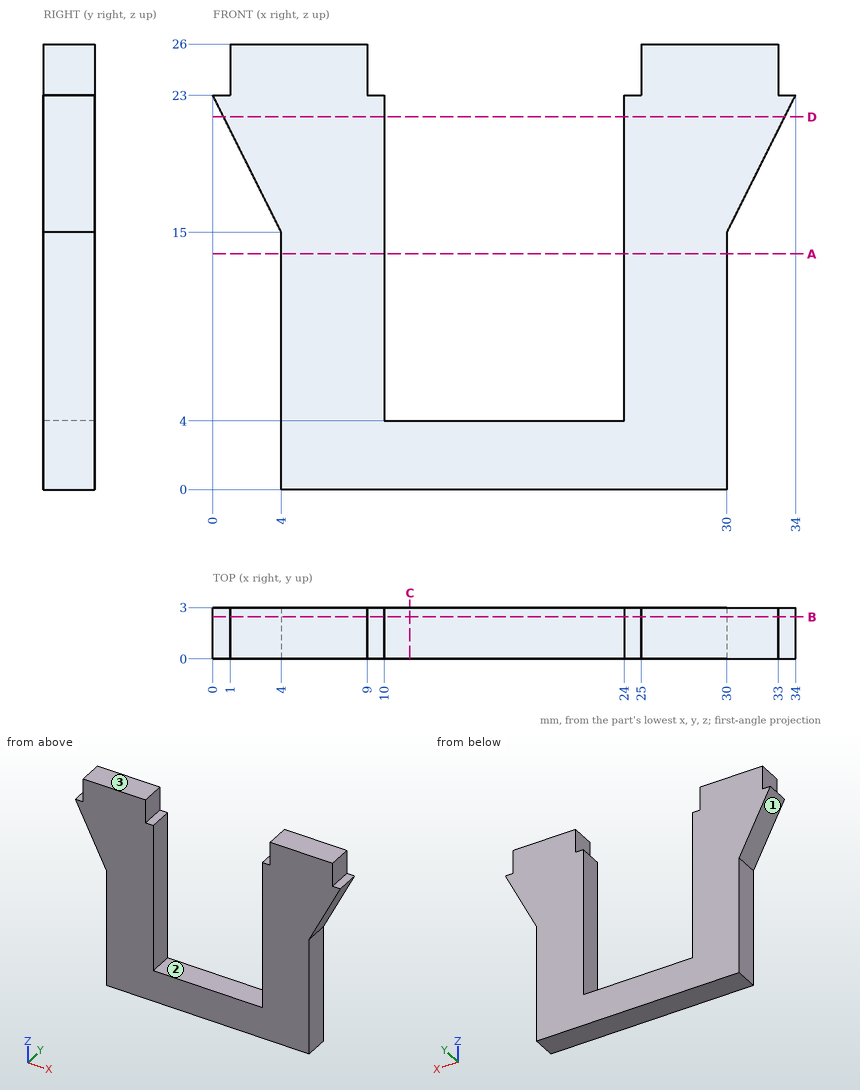
Geometry check sheet. Reference: drawing and pictorial views, mm from the part's lowest x, y, z. Coordinates: 2 decimals unless noted, no trailing zeros. Write each loop counter-clockwise with the first axis right and the second up, starting at its lowest first coordinate (ties: lowest second). Pieces come first, ordered by that corner, then holes.
Item 1: Cross-section at C-C on x = 11.5. Record the boundary of the cut face in (y, z).
Numbers:
outline: (0, 0) - (3, 0) - (3, 4) - (0, 4) - close
Item 2: Cross-section at B-B on y = 2.45. Record the boundary of the cut face in (x, z), then the cut area to 3 significant figures.
Numbers:
outline: (0, 23) - (4, 15) - (4, 0) - (30, 0) - (30, 15) - (34, 23) - (33, 23) - (33, 26) - (25, 26) - (25, 23) - (24, 23) - (24, 4) - (10, 4) - (10, 23) - (9, 23) - (9, 26) - (1, 26) - (1, 23) - close
area: 412 mm2
Item 3: Cross-section at D-D on z = 21.75. Record the boundary of the cut face in (x, y) (3 decimals), then the cut area to 4 significant figures.
Numbers:
outline: (0.625, 0) - (10, 0) - (10, 3) - (0.625, 3) - close; (24, 0) - (33.375, 0) - (33.375, 3) - (24, 3) - close
area: 56.25 mm2
Item 4: Depth check by flat-ended pin: pin 1 Ø1.5 at (y, z) = (2, 14.5) entering from +X (3 decimals); pin 2 Ø1.1 at (x, y) = (33.5, 2) entering from +Z; pin 3 Ø1.5 at (x, y) = (17.5, 1) entering from +Z; pin 4 Ø1 at (y, z) = (1.5, 8.5) entering from -X. Enter the tip coordinate at first touch or a pass-through.
Numbers:
pin 1: stops at x = 30.125
pin 2: stops at z = 26
pin 3: stops at z = 4
pin 4: stops at x = 4
Item 5: Scan lines: probe 1 along X at (y, z) = (2.5, 24); probe 2 along X at (y, z) = (1.05, 4.25); probe 3 along Z at (x, y) = (12, 1.3). Record each from-to range of solid material in increasing order.
Numbers:
probe 1: x = 1 to 9, 25 to 33
probe 2: x = 4 to 10, 24 to 30
probe 3: z = 0 to 4
Item 6: Mould release check, pull along X, two halves, no side actions. Record for the marked faces 1, 2 and 3: released by +X, released by -X, zero draft, split by the parting line, or undercut.
Numbers:
face 1: released by -X
face 2: undercut
face 3: zero draft
Item 7: Cross-section at A-A on z = 13.75. Record the boundary of the cut face in (x, y).
Numbers:
outline: (4, 0) - (10, 0) - (10, 3) - (4, 3) - close; (24, 0) - (30, 0) - (30, 3) - (24, 3) - close
